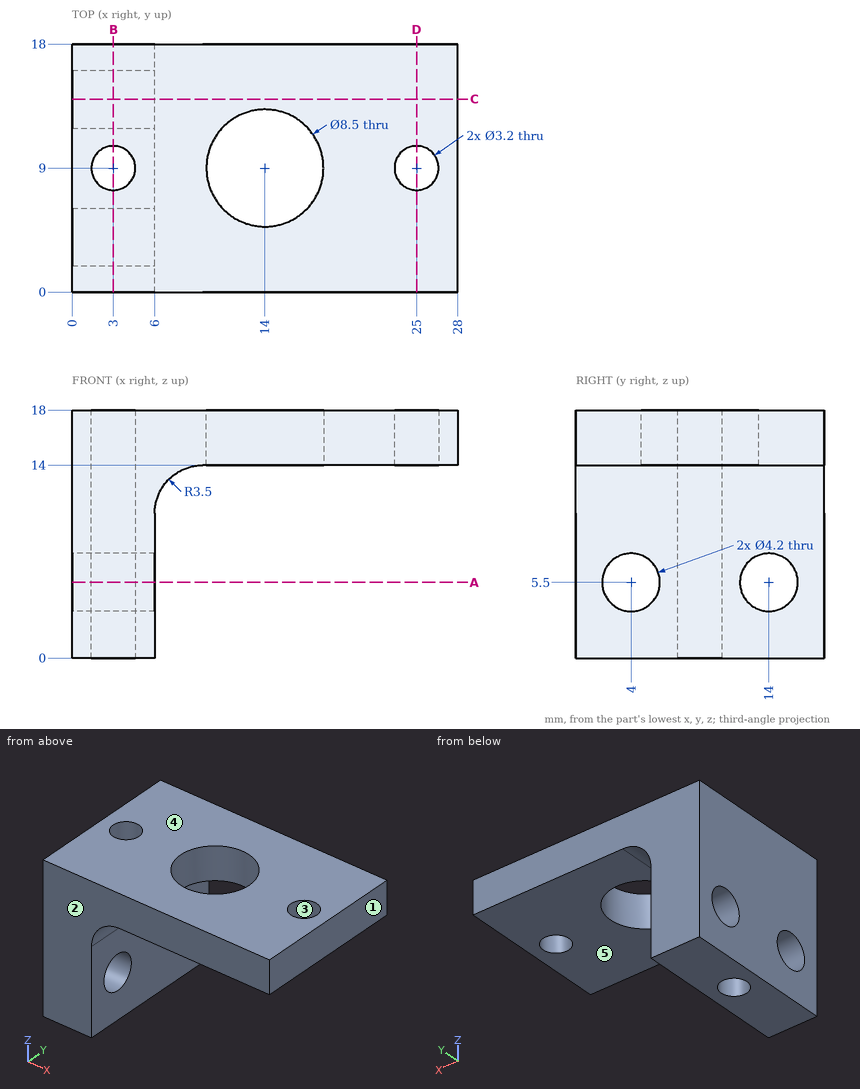
Could you check a few things on this drawing? It's one solid part, dimensions in mm from its lowest x, y, z. A direction names the side the tool comes from. Coordinates: 2 decimals unless noted, no trailing zeros. Write each loop counter-clockwise with the first axis right and the second up, starting at its lowest first coordinate (ties: lowest second). Pieces come first, ordered by that corner, then holes. Notation, with made-up numbers: (4, -25) - (22, -25) arc R7 cw to (22, -19) - close; hole circle Ø4 at (63, 37.25). An arc over 180 degrees is marked (long way). Put each result on its own line as item: value. Start each with the question number.
Q1. Which directions (+Z, -Z, +X, -X, +Y, -Y) give clear straight access to the entire face, cutting with the end or side of a thin tool? Please do the marked faces 4 and 5.
Q2. I want a section at A-A on z = 5.5. Write out the boundary of the cut face in (x, y), plus the area to 3 significant figures.
Q3. I want a section at C-C on y = 14. Write out the boundary of the cut face in (x, z).
Q4. I'm going to push flat-ended pins straight in: P1, Ø10, axis at x = 23, y = 6.5, coming from the -Z side; P2, Ø5, axis at x = 10, z = 12.5, coming from the -Y side; P3, Ø2.5, axis at y = 14, z = 5.5, coming from the -X side; P4, Ø5, axis at y = 4, z = 5.5, coming from the +X side. Where does each tip first touch, or does it pass through?
Q5. Thinking about a two-plate mould opening in X: for the marked faces 1, 2 and 3, which applies, pulls with the +X half, pulls with the -X half, needs draft (parallel to the pull), parting line crosses it, or undercut?
Q6. I want a section at D-D on x = 25. Write out the boundary of the cut face in (y, z), plus the area to 3 significant figures.
Q7. Please list where these lines run through material, in increasing order: L1, parallel to Y at x = 1.3, z = 5.5; L2, parallel to Y at x = 14, z = 14.85; L3, parallel to Y at x = 2.1, z = 5.5.
Q8. I want a section at B-B on x = 3. Write out the boundary of the cut face in (y, z).
Checks:
1. face 4: +Z, +X, -X, +Y, -Y
1. face 5: -Z, +X, +Y, -Y
2. outline: (0, 0) - (6, 0) - (6, 1.9) - (0, 1.9) - close; (0, 6.1) - (6, 6.1) - (6, 11.9) - (0, 11.9) - close; (0, 16.1) - (6, 16.1) - (6, 18) - (0, 18) - close; hole circle Ø3.2 at (3, 9)
2. area: 49.6 mm²
3. outline: (0, 0) - (6, 0) - (6, 3.4) - (0, 3.4) - close; (0, 7.6) - (6, 7.6) - (6, 10.5) arc R3.5 cw to (9.5, 14) - (28, 14) - (28, 18) - (0, 18) - close
4. P1: z = 14
4. P2: y = 0
4. P3: through
4. P4: x = 6
5. face 1: pulls with the +X half
5. face 2: needs draft
5. face 3: undercut
6. outline: (0, 14) - (7.4, 14) - (7.4, 18) - (0, 18) - close; (10.6, 14) - (18, 14) - (18, 18) - (10.6, 18) - close
6. area: 59.2 mm²
7. L1: 0 to 1.9, 6.1 to 11.9, 16.1 to 18
7. L2: 0 to 4.75, 13.25 to 18
7. L3: 0 to 1.9, 6.1 to 7.68, 10.32 to 11.9, 16.1 to 18
8. outline: (0, 0) - (7.4, 0) - (7.4, 18) - (0, 18) - close; (10.6, 0) - (18, 0) - (18, 18) - (10.6, 18) - close; hole circle Ø4.2 at (4, 5.5); hole circle Ø4.2 at (14, 5.5)
